The model under review builds one solid part; all positions refer to its coordinate system, in mm. Face numbers are marked on the shaded views. A direction names the side the tool comes from. Coordinates: 2 decimals unless noted, no trailing zeros. Loops run counter-clockwise (first coordinate to the right, second up) from the corner with the lowest first, then second, coordinate; pieces in that order, holes last. Notation, with made-up numbers: (-12.5, 14) - (35.5, 14) arc R13 ccw to (35.5, 21) - close; hole circle Ø10 at (-0.5, 67). An arc over 180 degrees is marked (long way). Use a Markdown table: item, result. Add a question column.
1) Add section B-B, the plane y = 0. Give the boundary of the cut face in (x, z), and give its area (4 significant figures).
2) For the marked faces 4 and 5, list the 3-axis set-ups (+Z, -Z, +X, -X, +Y, -Y) from which the entire face can be reached by the end or side of a thin tool; tool diameter is ignored.
3) To check wall thickness, follow L1, parallel to Y at x = 38.5, z = 7.4; L2, parallel to Y at x = -8.5, z = 2.2; L3, parallel to Y at x = 18, z = 2.25. State the ranges of each line that lie inside material, in increasing order. Write a range as [from, to].
4) The part is to be moulded in two halves that separate along X. For the marked faces 1, 2 and 3, say which applies: pulls with the +X half, pulls with the -X half, needs draft (parallel to the pull), parting line crosses it, or undercut.
5) Add section C-C, the plane x = -8.5. Give the boundary of the cut face in (y, z), and give its area (3 significant figures).
6) Add section A-A, the plane x = 15. Give the boundary of the cut face in (y, z), and give its area (3 significant figures).
7) Add section D-D, the plane z = 6. Give the boundary of the cut face in (x, y).
8) Clearance check with flat-ended pins moving along their axes: pin 1 (10 mm diameter, centred on x = -29, y = -13, fed in from -Z); pin 2 (5.5 mm diameter, centred on x = 38.5, y = 23.5, fed in from -Z) (1 decimal); pin 3 (7 mm diameter, centred on x = 38.5, y = -23.5, fed in from +Z). State where each tip first meets the part, or that it passes through.
```python
from build123d import *

# Parameters (mm, degrees)
F0_W           = 87
F0_H           = 57
F1_DEPTH       = 10
F2_R           = 19.25
F2_R_2         = 3
F2_R_3         = 3.5
F3_DEPTH       = 10.001
F5_R           = 5.5
F6_DEPTH       = 6
F7_D           = 6
F7_CBORE_D     = 9
F7_CBORE_DEPTH = 5.5
F8_R           = 5
F9_SIZE        = 5


with BuildPart() as f1:
    # F0 (on Top) → F1 (new body)
    with BuildSketch(Plane.XY):
        Rectangle(F0_W, F0_H)
    extrude(amount=F1_DEPTH)

    # F2 (on face) → F3 (cut, through all)
    with BuildSketch(Plane.XY.offset(10)):
        with Locations((15, 0)):
            Circle(F2_R)
        with Locations((-28.5, 13.5)):
            Circle(F2_R_2)
        with Locations((-28.5, -13.5)):
            Circle(F2_R_3)
    extrude(amount=-F3_DEPTH, mode=Mode.SUBTRACT)

    # F5 (on face) → F6 (cut)
    with BuildSketch(Plane.XY.offset(10)):
        with Locations((-28.5, 13.5)):
            Circle(F5_R)
        with Locations((-28.5, -13.5)):
            Circle(F5_R)
    extrude(amount=-F6_DEPTH, mode=Mode.SUBTRACT)

    # F7 (through all)
    with Locations(Plane.XY.offset(10)):
        with Locations((-8.5, 23.5), (38.5, 23.5), (38.5, -23.5), (-8.5, -23.5)):
            CounterBoreHole(F7_D / 2, F7_CBORE_D / 2, F7_CBORE_DEPTH)

    # F8
    f8_edges = [f1.edges().sort_by_distance(p)[0] for p in [
        (43.5, -28.5, 5),
        (43.5, 28.5, 5),
    ]]
    fillet(f8_edges, radius=F8_R)

    # F9
    f9_edges = [f1.edges().sort_by_distance(p)[0] for p in [
        (-43.5, 0, 10),
    ]]
    chamfer(f9_edges, length=F9_SIZE)


solid = f1.part
```
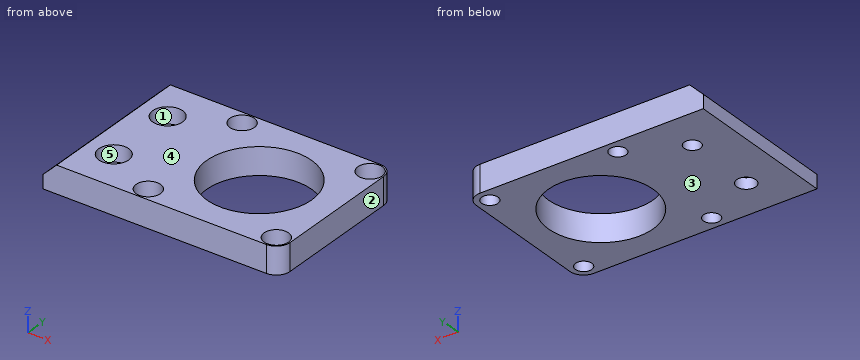
From the geometry:
| question | item | result |
|---|---|---|
| 1 | outline | (-43.5, 0) - (-4.25, 0) - (-4.25, 10) - (-38.5, 10) - (-43.5, 5) - close; (34.25, 0) - (43.5, 0) - (43.5, 10) - (34.25, 10) - close |
| 1 | area | 472.5 mm^2 |
| 2 | face 4 | +Z, +X, -X, +Y, -Y |
| 2 | face 5 | +Z |
| 3 | L1 | y = [-28.5, -28], [-19, 19], [28, 28.5] |
| 3 | L2 | y = [-28.5, -26.5], [-20.5, 20.5], [26.5, 28.5] |
| 3 | L3 | y = [-28.5, -19.01], [19.01, 28.5] |
| 4 | face 1 | undercut |
| 4 | face 2 | pulls with the +X half |
| 4 | face 3 | needs draft |
| 5 | outline | (-28.5, 0) - (-26.5, 0) - (-26.5, 4.5) - (-28, 4.5) - (-28, 10) - (-28.5, 10) - close; (-20.5, 0) - (20.5, 0) - (20.5, 4.5) - (19, 4.5) - (19, 10) - (-19, 10) - (-19, 4.5) - (-20.5, 4.5) - close; (26.5, 0) - (28.5, 0) - (28.5, 10) - (28, 10) - (28, 4.5) - (26.5, 4.5) - close |
| 5 | area | 417 mm^2 |
| 6 | outline | (-28.5, 0) - (-19.25, 0) - (-19.25, 10) - (-28.5, 10) - close; (19.25, 0) - (28.5, 0) - (28.5, 10) - (19.25, 10) - close |
| 6 | area | 185 mm^2 |
| 7 | outline | (-42.5, -28.5) - (38.5, -28.5) arc R5 ccw to (43.5, -23.5) - (43.5, 23.5) arc R5 ccw to (38.5, 28.5) - (-42.5, 28.5) - close; hole circle Ø11 at (-28.5, -13.5); hole circle Ø11 at (-28.5, 13.5); hole circle Ø9 at (-8.5, -23.5); hole circle Ø9 at (-8.5, 23.5); hole circle Ø38.5 at (15, 0); hole circle Ø9 at (38.5, -23.5); hole circle Ø9 at (38.5, 23.5) |
| 8 | pin 1 | stops at z = 0 |
| 8 | pin 2 | passes through |
| 8 | pin 3 | stops at z = 4.5 |
